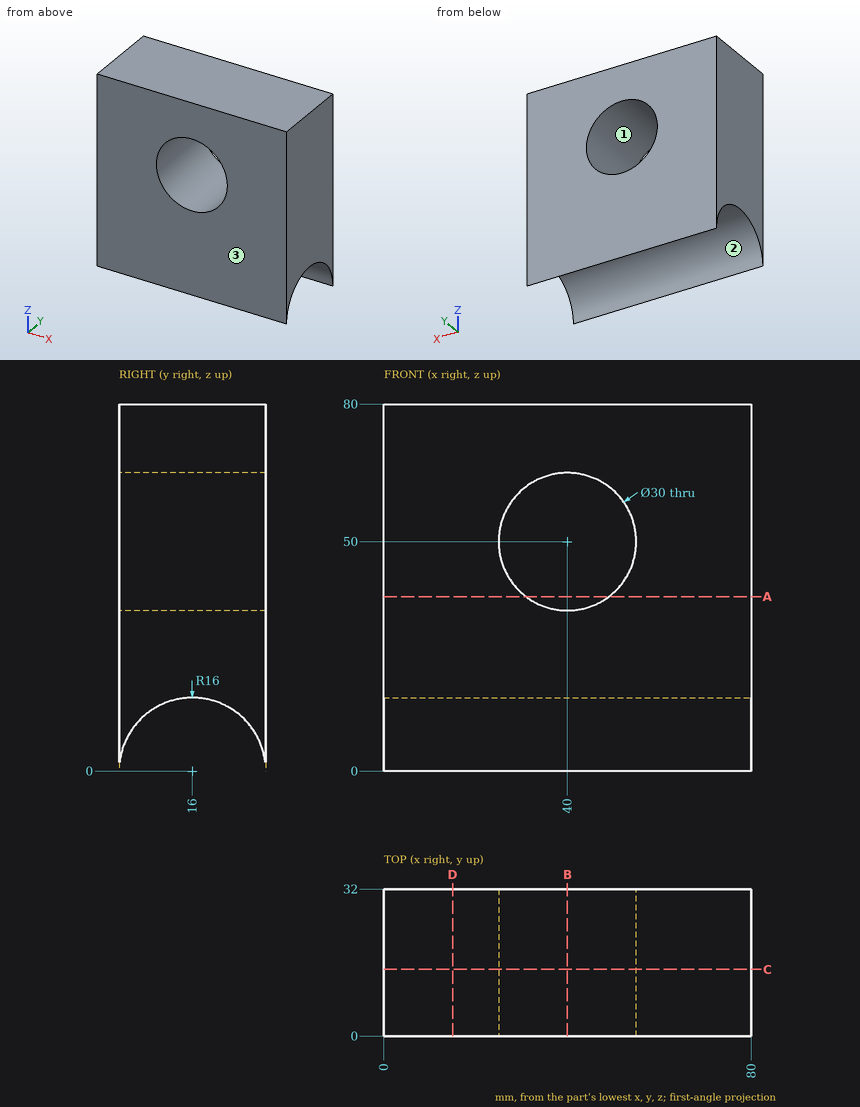
Check sheet for the drawn part. Datum: minimum x, y, z corner. Units: mm. Coordinates: 2 decimals unless noted, no trailing zeros. Write each loop counter-clockwise with the first axis right and the second up, starting at its lowest first coordinate (ties: lowest second). Pieces come first, ordered by that corner, then holes. Notation, with made-up numbers: M 22,-13.5 L 34,-13.5 A24 ccw 34,13.5 Z; hole C 79,70 d7. An arc over 180 degrees is marked long. One line per item, written item: value.
Item 1: Section check B-B, the plane x = 40. Record the boundary of the cut face in (y, z), plus the area to 3 significant figures.
Check sheet entries:
outline: M 0,0 A16 cw 32,0 L 32,35 L 0,35 Z; M 0,65 L 32,65 L 32,80 L 0,80 Z
area: 1,200 mm^2
Item 2: Section check D-D, the plane x = 15. Record the boundary of the cut face in (y, z).
Check sheet entries:
outline: M 0,0 A16 cw 32,0 L 32,80 L 0,80 Z
Item 3: Scan lines: line 1 along Z through (x, y) = (35, 4.5); line 2 along X through (y, z) = (3.5, 59); line 3 along Y through (x, z) = (46.5, 9.5). Record each from-to range of solid material in increasing order.
Check sheet entries:
line 1: z = 11.12 to 35.86, 64.14 to 80
line 2: x = 0 to 28, 52 to 80
line 3: y = 0 to 3.13, 28.87 to 32
Item 4: Mould release check, pull along Y, two halves, no side actions. Record for the marked faces 1, 2 and 3: pulls with the +Y half, pulls with the -Y half, needs draft (parallel to the pull), parting line crosses it, or undercut.
Check sheet entries:
face 1: needs draft
face 2: undercut
face 3: pulls with the -Y half
Item 5: Gauge pin test, flat ends, axial feed: pin 1 Ø1 at (x, y) = (34.5, 20.5) entering from -Z; pin 2 Ø2 at (x, y) = (63, 4) entering from -Z; pin 3 Ø2 at (x, y) = (70, 16) entering from -Z. Record the tip position at first contact, or that the pin passes through.
Check sheet entries:
pin 1: stops at z = 15.2
pin 2: stops at z = 9.33
pin 3: stops at z = 15.97
Item 6: Section check C-C, the plane y = 14.5. Record the boundary of the cut face in (x, z).
Check sheet entries:
outline: M 0,15.93 L 80,15.93 L 80,80 L 0,80 Z; hole C 40,50 d30
Item 7: Section check A-A, the plane z = 38. Record the boundary of the cut face in (x, y), plus the area to 3 significant figures.
Check sheet entries:
outline: M 0,0 L 31,0 L 31,32 L 0,32 Z; M 49,0 L 80,0 L 80,32 L 49,32 Z
area: 1,980 mm^2
